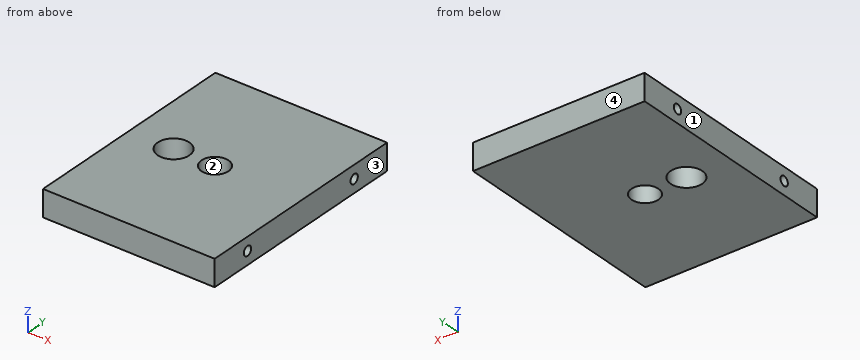
```python
from build123d import *

# Parameters (mm, degrees)
SKETCH1_W                 = 32.5
SKETCH1_H                 = 42
BOSS_EXTRUDE2_DEPTH       = 5
F_2_56_TAPPED_HOLE1_D     = 1.778
F_2_56_TAPPED_HOLE1_DEPTH = 7.46583491
F_2_56_TAPPED_HOLE1_TIP   = 0.53416509
F_2_56_TAPPED_HOLE2_D     = 1.778
F_2_56_TAPPED_HOLE2_DEPTH = 7.46583491
F_2_56_TAPPED_HOLE2_TIP   = 0.53416509
CUT_EXTRUDE1_DEPTH        = 5
F_1_4_20_TAPPED_HOLE1_D   = 5.1054


with BuildPart() as part:
    # Sketch1 → Boss-Extrude2 (new body)
    with BuildSketch(Plane.XY):
        with Locations((16.25, 21)):
            Rectangle(SKETCH1_W, SKETCH1_H)
    extrude(amount=BOSS_EXTRUDE2_DEPTH)

    # #2-56 Tapped Hole1
    with Locations(Plane.ZY):
        with Locations((2.5, 34), (2.5, 8)):
            Hole(F_2_56_TAPPED_HOLE1_D / 2, depth=F_2_56_TAPPED_HOLE1_DEPTH)
            with Locations((0, 0, -(F_2_56_TAPPED_HOLE1_DEPTH + F_2_56_TAPPED_HOLE1_TIP / 2))):  # 118° drill point
                Cone(0, F_2_56_TAPPED_HOLE1_D / 2, F_2_56_TAPPED_HOLE1_TIP, mode=Mode.SUBTRACT)

    # #2-56 Tapped Hole2
    with Locations(Plane(origin=(32.5, 0, 0), x_dir=(0, 0, -1), z_dir=(1, 0, 0))):
        with Locations((-2.5, 34), (-2.5, 8)):
            Hole(F_2_56_TAPPED_HOLE2_D / 2, depth=F_2_56_TAPPED_HOLE2_DEPTH)
            with Locations((0, 0, -(F_2_56_TAPPED_HOLE2_DEPTH + F_2_56_TAPPED_HOLE2_TIP / 2))):  # 118° drill point
                Cone(0, F_2_56_TAPPED_HOLE2_D / 2, F_2_56_TAPPED_HOLE2_TIP, mode=Mode.SUBTRACT)

    # Sketch9 → Cut-Extrude1 (cut)
    with BuildSketch(Plane(origin=(0, 0, 0), x_dir=(-1, 0, 0), z_dir=(0, 0, -1))):
        with BuildLine():
            ThreePointArc((-11.4, 21), (-8.4, 18), (-5.4, 21))
            Line((-5.4, 21), (-8.4, 21))
            Line((-8.4, 21), (-11.4, 21))
        make_face()
        with BuildLine():
            Line((-8.4, 21), (-5.4, 21))
            ThreePointArc((-5.4, 21), (-8.4, 24), (-11.4, 21))
            Line((-11.4, 21), (-8.4, 21))
        make_face()
    extrude(amount=-CUT_EXTRUDE1_DEPTH, mode=Mode.SUBTRACT)

    # 1/4-20 Tapped Hole1 (through all)
    with Locations(Plane(origin=(0, 0, 0), x_dir=(-1, 0, 0), z_dir=(0, 0, -1))):
        with Locations((-16.25, 21)):
            Hole(F_1_4_20_TAPPED_HOLE1_D / 2)


solid = part.part
```
Can you work these out from the model? Positions are in its coordinate system, mm. Face numbers are marked on the shaded views. Give positions to 0.01 mm unless a question says otherwise; leave off trailing zeros. Loops run counter-clockwise (first coordinate to the right, second up) from the corner with the lowest first, then second, coordinate; pieces in that order, holes last. Notation, with made-up numbers: M 16.25,4.25 L 43.25,4.25 A17 cw 43.25,33.25 Z; hole C 7,21 d6. An arc over 180 degrees is marked long. One line per question, with ' | ' between items. Start each with the question number.
Q1. For pin 1 Ø1.5 at (x, z) = (14, 2) entering from -Y; pin 2 Ø1.1 at (y, z) = (8, 2.5) entering from -X; pin 3 Ø1.4 at (y, z) = (34, 2.5) entering from -X, each with a flat end and sliding along its axis, tell me the tip position at first contact or that it passes through.
Q2. If we section it at A-A (y = 21): Please give me the cut outline in (x, z).
Q3. If we section it at B-B (x = 16.25): Please give me the cut outline in (y, z), plus the area to 3 significant figures.
Q4. If I drill on line 1 (Y direction, x = 4, z = 2.5); line 2 (Z direction, x = 4.5, y = 34); line 3 (Y direction, x = 30.5, z = 2.8), over which ranges is the centre line in solid material (lowest first)? Write a range as from..to.
Q5. If we section it at D-D (x = 26): Please give me the cut outline in (y, z).
Q6. If we mould it in two halves opening along X, with no side actions, what happens to the marked faces 1, 2, 3 and 4? For each: +X half, -X half, draft (parallel to the pull), parting line (faces both ways), or undercut.
Q7. If we section it at C-C (z = 4.3): Please give me the cut outline in (x, y).
Computed:
1) pin 1: stops at y = 0 | pin 2: stops at x = 7.67 | pin 3: stops at x = 7.58
2) outline: M 0,0 L 5.4,0 L 5.4,5 L 0,5 Z; M 11.4,0 L 13.7,0 L 13.7,5 L 11.4,5 Z; M 18.8,0 L 32.5,0 L 32.5,5 L 18.8,5 Z
3) outline: M 0,0 L 18.45,0 L 18.45,5 L 0,5 Z; M 23.55,0 L 42,0 L 42,5 L 23.55,5 Z | area: 184 mm²
4) line 1: y = 0..7.11, 8.89..33.11, 34.89..42 | line 2: z = 0..1.61, 3.39..5 | line 3: y = 0..7.16, 8.84..33.16, 34.84..42
5) outline: M 0,0 L 42,0 L 42,5 L 0,5 Z; hole C 8,2.5 d1.78; hole C 34,2.5 d1.78
6) face 1: -X half | face 2: undercut | face 3: +X half | face 4: draft
7) outline: M 0,0 L 32.5,0 L 32.5,42 L 0,42 Z; hole C 8.4,21 d6; hole C 16.25,21 d5.11
